The model under review builds one solid part; all positions refer to its coordinate system, in mm. A direction names the side the tool comes from. Coordinates: 2 decimals unless noted, no trailing zeros. Write each loop counter-clockwise with the first axis right and the second up, starting at its lowest first coordinate (ties: lowest second). Pieces come first, ordered by that corner, then holes.
```python
from build123d import *

# Parameters (mm, degrees)
SKETCH2_R           = 4
BOSS_EXTRUDE1_DEPTH = 2.5
SKETCH2_6_R         = 4
SKETCH2_6_R_2       = 2.5
BOSS_EXTRUDE2_DEPTH = 2.5
SKETCH3_R           = 2.5
BOSS_EXTRUDE3_DEPTH = 14.5
CHAMFER2_SIZE       = 1
CUT_EXTRUDE1_DEPTH  = 1.5


with BuildPart() as part:
    # Sketch2 → Boss-Extrude1 (new body)
    with BuildSketch(Plane.XY):
        Circle(SKETCH2_R)
    extrude(amount=BOSS_EXTRUDE1_DEPTH)

    # Sketch2<6> → Boss-Extrude2 (add)
    with BuildSketch(Plane.XY):
        Circle(SKETCH2_6_R)
        Circle(SKETCH2_6_R_2, mode=Mode.SUBTRACT)
    extrude(amount=BOSS_EXTRUDE2_DEPTH)

    # Sketch3 → Boss-Extrude3 (add)
    with BuildSketch(Plane.XY.offset(2.5)):
        with Locations(Location((0, 0, 0), (0, 0, 180))):
            Circle(SKETCH3_R)
    extrude(amount=BOSS_EXTRUDE3_DEPTH)

    # Chamfer2
    chamfer2_edges = [part.edges().sort_by_distance(p)[0] for p in [
        (-4, 0, 0),
    ]]
    chamfer(chamfer2_edges, length=CHAMFER2_SIZE)

    # Sketch4 → Cut-Extrude1 (cut)
    with BuildSketch(Plane(origin=(0, 0, 0), x_dir=(-1, 0, 0), z_dir=(0, 0, -1))):
        Polygon((-0.870420924, 2.834447623), (-2.889914109, 0.66341718), (-2.019493185, -2.171030443), (0.870420924, -2.834447623), (2.889914109, -0.66341718), (2.019493185, 2.171030443), align=None)
    extrude(amount=-CUT_EXTRUDE1_DEPTH, mode=Mode.SUBTRACT)


solid = part.part
```
Item 1: Machinability: for faces 4 (the face through (0, 0, 17)), 5 (the face through (2.5, -0.1, 9.6)), 6 (the face through (0, 0, 1.5)), which of the approach directions +Z, -Z, +X, -X, +Y, -Y give a long, thin tool a straight path to every point of the face, cutting with its end or side? Answer none if there is none.
Solved:
face 4: +Z, +X, -X, +Y, -Y
face 5: +Z
face 6: -Z
Item 2: Take a section at B-B, the plane x = 0. Write out the cut boundary in (y, z).
Solved:
outline: (-4, 1) - (-3, 0) - (-2.63, 0) - (-2.63, 1.5) - (2.63, 1.5) - (2.63, 0) - (3, 0) - (4, 1) - (4, 2.5) - (2.5, 2.5) - (2.5, 17) - (-2.5, 17) - (-2.5, 2.5) - (-4, 2.5) - close
Item 3: Take a section at A-A, the plane z = 6.5. Write out the cut boundary in (x, y).
Solved:
outline: circle Ø5 at (0, 0)
Item 4: For pin 1 (1 mm diameter, centred on x = -1, z = 9.5, fed in from -Y); pin 2 (4 mm diameter, centred on x = -1, z = 13, fed in from +Y); pin 3 (2 mm diameter, centred on y = 2.5, z = 4, fed in from +X), all flat-tipped, find the tip position at first contact; note any pin that passes through.
Solved:
pin 1: stops at y = -2.45
pin 2: stops at y = 2.5
pin 3: stops at x = 2
Item 5: Take a section at C-C, the plane y = 0. Write out the cut boundary in (x, z).
Solved:
outline: (-4, 1) - (-3, 0) - (-2.69, 0) - (-2.69, 1.5) - (2.69, 1.5) - (2.69, 0) - (3, 0) - (4, 1) - (4, 2.5) - (2.5, 2.5) - (2.5, 17) - (-2.5, 17) - (-2.5, 2.5) - (-4, 2.5) - close
Item 6: To check wall thickness, follow line 1 along Z through (x, y) = (0, -2.25); line 2 along Z through (x, y) = (3, 2.25); line 3 along Y through (x, z) = (1.75, 4.75). State the ranges of each line that lie inside material, in increasing order.
Solved:
line 1: z = 1.5 to 17
line 2: z = 0.75 to 2.5
line 3: y = -1.79 to 1.79
Item 7: Mouldability with a two-part tool opening along X and no side actions: class faces 1 (the face through (2, 2, 0)), 2 (the face through (0.59, -2.5, 0.74)), 3 (the face through (-0.867, -3.905, 1.74)) as pulls with the +X half, pulls with the -X half, needs draft (parallel to the pull), parting line crosses it, or undercut.
Solved:
face 1: needs draft
face 2: undercut
face 3: parting line crosses it
